from build123d import *

# Parameters (mm, degrees)
SKETCH_1_W          = 10
SKETCH_1_H          = 10
SKETCH_1_W_2        = 8
SKETCH_1_H_2        = 8
EXTRUDE_1_DEPTH     = 214.97
SKETCH_2_R          = 1.6
CUT_EXTRUDE_1_DEPTH = 213.715


with BuildPart() as part:
    # ｽｹｯﾁ1 → ﾎﾞｽ - 押し出し1 (new, symmetric)
    with BuildSketch(Plane(origin=(0, 0, 0), x_dir=(1, 0, 0), z_dir=(0, 1, 0))):
        Rectangle(SKETCH_1_W, SKETCH_1_H)
        Rectangle(SKETCH_1_W_2, SKETCH_1_H_2, mode=Mode.SUBTRACT)
    extrude(amount=EXTRUDE_1_DEPTH, both=True)

    # ｽｹｯﾁ2 → ｶｯﾄ - 押し出し1 (cut, symmetric)
    with BuildSketch(Plane.XY.offset(5)):
        with Locations((0, 209.97)):
            Circle(SKETCH_2_R)
        with Locations((0, 189.97)):
            Circle(SKETCH_2_R)
    cut_extrude_1 = extrude(amount=CUT_EXTRUDE_1_DEPTH, both=True, mode=Mode.SUBTRACT)

    # ﾐﾗｰ1: ｶｯﾄ - 押し出し1 across plane
    add(cut_extrude_1.mirror(Plane.ZX), mode=Mode.SUBTRACT)


solid = part.part
Verification items for the finished model (mm, model axes). A direction names the side the tool comes from. Coordinates: 2 decimals unless noted, no trailing zeros. Loops run counter-clockwise (first coordinate to the right, second up) from the corner with the lowest first, then second, coordinate; pieces in that order, holes last. Notation, with made-up numbers: (-27.75, 53) -> (-22.75, 53) arc R28 cw to (-22.75, 90) -> close; hole circle Ø10 at (38.5, -38). An arc over 180 degrees is marked (long way). Answer as a JSON object with one key per item and string values. Group by question number.
Item 1: Scan lines: probe 1 along Y at (x, z) = (0, -4.5); probe 2 along X at (y, z) = (-49.5, 1). Record each from-to range of solid material in increasing order.
Item 2: Sectioned sample at A-A on y = 151. Record the boundary of the cut face in (x, z).
Item 3: Tool access check on faces 1 (the flat face through (0, 3, 5)), 2 (the flat face through (4, 3, 0)). Record the directions out of +Z, -Z, +X, -X, +Y, -Y that give a thin tool (end or side, any length) a straight path to the whole face; none if there is none.
Item 4: Sectioned sample at C-C on x = 0. State how many separate pieces and enclosed holes the cut face has, plus the area to 3 significant figures.
Item 5: Mould release check, pull along Z, two halves, no side actions. Record for faces 3 (the flat face through (0, 3, -4)), 4 (the flat face through (-5, 3, 0)), 5 (the flat face through (0, 3, 4)), 6 (the flat face through (0, 3, -5)): +Z half, -Z half, draft (parallel to the pull), parting line (faces both ways), or undercut.
Item 6: Sectioned sample at B-B on z = 1.75. Record the boundary of the cut face in (x, y), plus the area to 3 significant figures.
Evaluation:
{
 "1": {"probe 1": "y = -214.97 to -211.57, -208.37 to -191.57, -188.37 to 188.37, 191.57 to 208.37, 211.57 to 214.97", "probe 2": "x = -5 to -4, 4 to 5"},
 "2": {"outline": "(-5, -5) -> (5, -5) -> (5, 5) -> (-5, 5) -> close; hole (-4, -4) -> (4, -4) -> (4, 4) -> (-4, 4) -> close"},
 "3": {"face 1": "+Z, +X, -X, +Y, -Y", "face 2": "+Y, -Y"},
 "4": {"separate pieces": "10", "enclosed holes": "0", "area": "834 mm²"},
 "5": {"face 3": "undercut", "face 4": "draft", "face 5": "undercut", "face 6": "-Z half"},
 "6": {"outline": "(-5, -214.97) -> (-4, -214.97) -> (-4, 214.97) -> (-5, 214.97) -> close; (4, -214.97) -> (5, -214.97) -> (5, 214.97) -> (4, 214.97) -> close", "area": "860 mm²"}
}
